Could you check a few things on this drawing? It's one solid part, dimensions in mm from its lowest x, y, z. Coordinates: 2 decimals unless noted, no trailing zeros. Write each loop counter-clockwise with the first axis right and the second up, starting at its lowest first coordinate (ties: lowest second). Pieces come first, ordered by that corner, then holes.
Item 1: Please list where these lines run through material, in increasing order: line 1 (X direction, y = 45.5, z = 10.5) (1 decimal); line 2 (Y direction, x = 102.5, z = 10.75); line 3 (Y direction, x = 66.5, z = 19.25) (1 decimal).
Item 2: I want a section at A-A (z = 10.25). Please give me the cut outline in (x, y) (1 decimal), and give its area (3 significant figures).
Item 3: I'm going to push flat-ended pins straight in: P1, Ø10, axis at y = 204.5, z = 10.5, coming from the -X side (1 decimal); P2, Ø1, axis at x = 183, z = 17, coming from the -Y side (1 decimal); P3, Ø6, axis at x = 257, z = 19.5, coming from the -Y side (1 decimal). Where does each tip first touch, or does it pass through?
Item 4: I want a section at B-B (x = 327.5). Please give me the cut outline in (y, z) (1 decimal).
Item 5: I want a section at C-C (y = 42). Please give me the cut outline in (x, z), and give its area (3 significant figures).
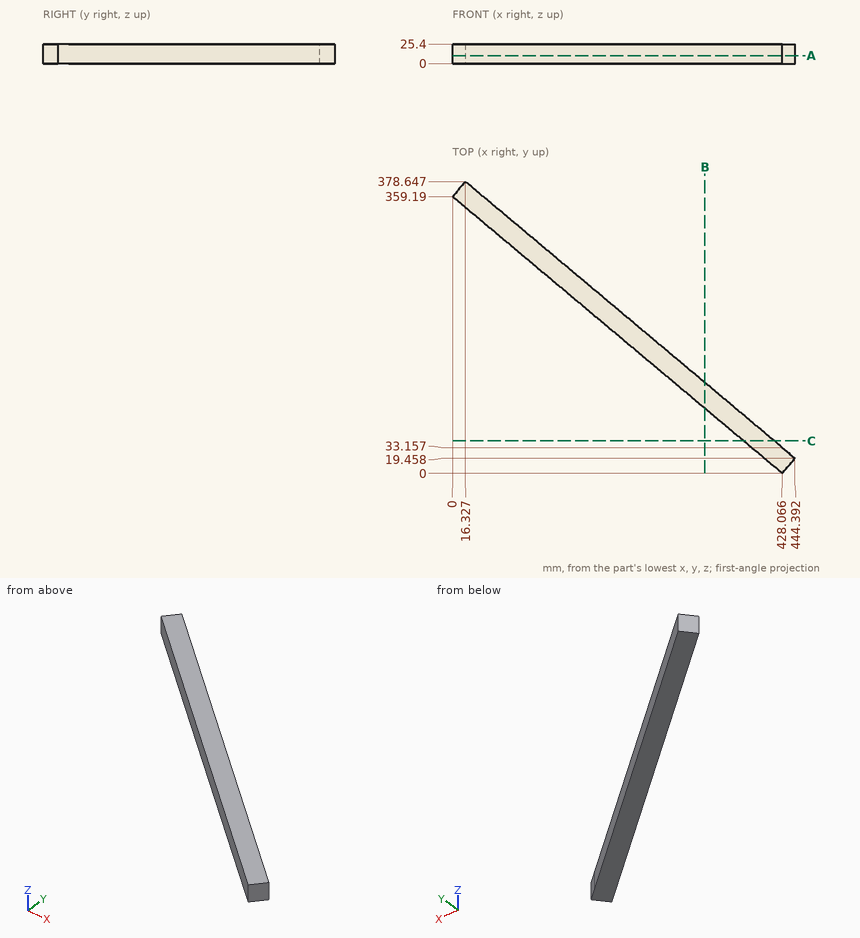
Answer:
1. line 1: x = 373.8 to 413.4
1. line 2: y = 273.18 to 306.34
1. line 3: y = 303.4 to 336.5
2. outline: (0, 359.2) - (428.1, 0) - (444.4, 19.5) - (428.1, 33.2) - (16.3, 378.6) - close
2. area: 14,200 mm2
3. P1: stops at x = 178.4
3. P2: stops at y = 205.2
3. P3: stops at y = 141
4. outline: (84.4, 0) - (117.5, 0) - (117.5, 25.4) - (84.4, 25.4) - close
5. outline: (378.01, 0) - (417.53, 0) - (417.53, 25.4) - (378.01, 25.4) - close
5. area: 1,000 mm2
